Autodesk Inventor part; units mm, degrees
ref_plane "YZ Plane" through (0, 0, 0) normal (1, 0, 0) x (0, 1, 0)
ref_plane "XZ Plane" through (0, 0, 0) normal (0, 1, 0) x (-1, 0, 0)
ref_plane "XY Plane" through (0, 0, 0) normal (0, 0, 1) x (1, 0, 0)
sketch "Sketch1" plane through (0, 0, 0) normal (0, 0, 1) x (1, 0, 0)
  circle A0 centre (0, 0) radius 9.525
  line L0 (0, 0) -> (0, 15.875)
  circle A1 centre (0, 15.875) radius 1.905
  circle A2 centre (-15.875, 0) radius 1.905
  circle A3 centre (0, -15.875) radius 1.905
  circle A4 centre (15.875, 0) radius 1.905
  circle A5 centre (0, 0) radius 20.6375
  dimension "d0" = 19.05
  dimension "d1" = 15.875
  dimension "d2" = 3.81
  dimension "d5" = 360
  dimension "d7" = 41.275
extrude "Extrusion1" add sketch "Sketch1" against normal blind 1.905
chamfer "Chamfer1" distance 1.27 angle 45 4 edges at (-1.905, 15.875, 0) (13.97, 0, 0) (-1.905, -15.875, 0) (-17.78, 0, 0)
sketch "Sketch4" plane through (0, 0, 0) normal (0, 0, 1) x (1, 0, 0)
  circle A0 centre (0, -15.875) radius 3.175
  circle A1 centre (0, 15.875) radius 3.175
  circle A2 centre (0, 0) radius 9.525
  circle A3 centre (0, 0) radius 20.6375
  circle A4 centre (15.875, 0) radius 3.175
  circle A5 centre (-15.875, 0) radius 3.175
extrude "Extrusion3" add sketch "Sketch4" along normal blind 2.032
sketch "Sketch5" plane through (0, 0, 2.032) normal (0, 0, 1) x (1, 0, 0)
  circle A0 centre (0, 0) radius 11.43
  dimension "d17" = 22.86
extrude "Extrusion4" cut sketch "Sketch5" against normal blind 2.032
properties part number "RadialBearingMountCover"
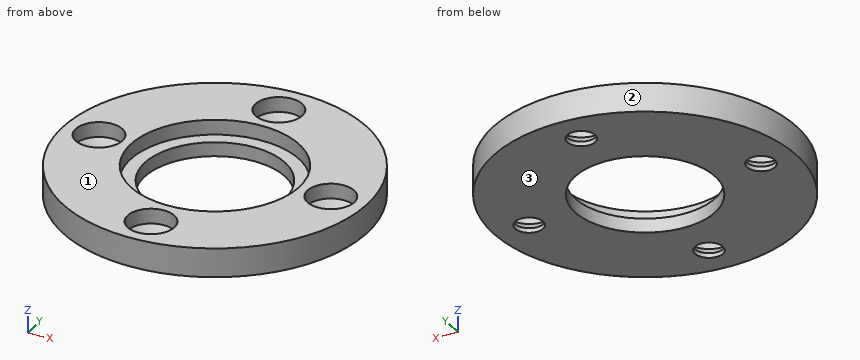
Read the model definition and answer for the solid it produces. Units are mm, in the model's axes. Face numbers are marked on the shaded views. Coordinates: 2 decimals unless noted, no trailing zeros. Loops run counter-clockwise (first coordinate to the right, second up) from the corner with the lowest first, then second, coordinate; pieces in that order, holes last. Notation, with made-up numbers: (6.25, 84) - (24.25, 84) arc R29 ccw to (24.25, 108) - close; hole circle Ø5 at (36.5, 74.5). An arc over 180 degrees is marked (long way). Answer in a Markdown table with one row per item.
Q1. Given P1, Ø5.5, axis at x = 15.875, y = 0, coming from the +Z side (3 decimals); P2, Ø1.5, axis at x = -13.5, z = -0.5, coming from the -Y side; P3, Ø6, axis at x = 15.875, y = 0, coming from the +Z side (3 decimals), each flat-ended and moving along its own axis, determine where each tip first touches the part or whether it passes through.
Here are the results:
| item | result |
|---|---|
| P1 | stops at z = -0.425 |
| P2 | stops at y = -16.23 |
| P3 | stops at z = -0.175 |
Q2. Straight lines are drawn through the part: line 1 along Y through (x, z) = (0, -1.75) (1 decimal); line 2 along Y through (x, z) = (0, 0.15); line 3 along X through (y, z) = (13.5, 1.4). For each, find the intervals that lie inside material, in ascending order. Write a range as [from, to].
Here are the results:
| item | result |
|---|---|
| line 1 | y = [-20.6, -17.8], [-14, -9.5], [9.5, 14], [17.8, 20.6] |
| line 2 | y = [-20.64, -19.05], [-12.7, -11.43], [11.43, 12.7], [19.05, 20.64] |
| line 3 | x = [-15.61, -2.11], [2.11, 15.61] |
Q3. Find section A-A on y = 0. Count the separate pieces of the cut face and the enclosed holes in it, plus the area to 3 significant figures.
Here are the results:
| item | result |
|---|---|
| separate pieces | 4 |
| enclosed holes | 0 |
| area | 36.2 mm^2 |
Q4. Find section C-C on x = 9. Write down the section's boundary in (y, z) (3 decimals).
Here are the results:
| item | result |
|---|---|
| outline | (-18.572, -1.905) - (-3.119, -1.905) - (-3.119, 0) - (-7.046, 0) - (-7.046, 2.032) - (-18.572, 2.032) - close; (3.119, -1.905) - (18.572, -1.905) - (18.572, 2.032) - (7.046, 2.032) - (7.046, 0) - (3.119, 0) - close |
Q5. The mould has two halves that part along Z. Classify the marked faces 1, 2 and 3: pulls with the +Z half, pulls with the -Z half, needs draft (parallel to the pull), parting line crosses it, or undercut.
Here are the results:
| item | result |
|---|---|
| face 1 | pulls with the +Z half |
| face 2 | needs draft |
| face 3 | pulls with the -Z half |
